```python
from build123d import *

# Parameters (mm, degrees)
F0_R     = 1.5
F1_DEPTH = 20
F2_SIZE  = 0.5
F0_R_2   = 2.75
F3_DEPTH = 2.5
F4_SIZE  = 0.25
F6_DEPTH = 1.3


with BuildPart() as f1:
    # F0 (on Top) → F1 (new body)
    with BuildSketch(Plane.XY):
        Circle(F0_R)
    extrude(amount=-F1_DEPTH)

    # F2
    f2_edges = [f1.edges().sort_by_distance(p)[0] for p in [
        (-1.5, 0, -20),
    ]]
    chamfer(f2_edges, length=F2_SIZE)

    # F0 (on Top) → F3 (join)
    with BuildSketch(Plane.XY):
        Circle(F0_R_2)
        Circle(F0_R, mode=Mode.SUBTRACT)
        Circle(F0_R)
    extrude(amount=F3_DEPTH)

    # F4
    f4_edges = [f1.edges().sort_by_distance(p)[0] for p in [
        (-2.75, 0, 2.5),
        (-2.75, 0, 0),
    ]]
    chamfer(f4_edges, length=F4_SIZE)

    # F5 (on face) → F6 (cut)
    with BuildSketch(Plane.XY.offset(2.5)):
        Polygon((0.75963, -1.281313), (1.489464, 0.017202), (0.729835, 1.298515), (-0.75963, 1.281313), (-1.489464, -0.017202), (-0.729835, -1.298515), align=None)
    extrude(amount=-F6_DEPTH, mode=Mode.SUBTRACT)


solid = f1.part
```
The listing builds one solid part. Answer for the finished solid, in the listing's coordinates (mm). A direction names the side the tool comes from. Give positions to 0.01 mm unless a question says otherwise; leave off trailing zeros. Order: outer loops, then holes, each group sorted by start corner. A loop starts at its lowest first (then second) coordinate and runs counter-clockwise, first axis right, second up. Notation, with made-up numbers: M 14,52 L 20,52 A23 cw 20,68 Z; hole C -11,55 d4. An arc over 180 degrees is marked long. Put each result on its own line as item: value. Start each with the question number.
Item 1: The part is cut by section A-A, the plane z = 1. Determine the outline of the cut face in (x, y), and give its area (3 significant figures).
Item 2: The part is cut by section B-B, the plane x = 0. Determine the outline of the cut face in (y, z).
Item 3: Flat-ended cylindrical pins translate along their axes: P1, Ø1.3, axis at x = 0, y = 0.5, coming from the +Z side; P2, Ø2, axis at x = 0, z = -4.5, coming from the +Y side; P3, Ø1.5, axis at y = 1, z = -8, coming from the -X side. Find the tip coordinate at first contact, or state that the pin passes through.
Item 4: The part is cut by section C-C, the plane z = -16.75. Determine the outline of the cut face in (x, y), and give its area (3 significant figures).
Item 5: Which of the six approach directions +Z, -Z, +X, -X, +Y, -Y give full straight-line access (tool end or side, diameter ignored) to faces 5 (the face through (0, 0, -20)), 6 (the face through (0, -2, 0)), 7 (the face through (-1.115, -0.649, 1.859))?
Item 6: For a pull along X with two mould halves and no side action, classify faces 1 (the face through (1.12, -0.64, 1.86)), 2 (the face through (-1.5, 0.07, -9.61)), 3 (the face through (0, 0, 1.2)), 4 (the face through (1.1, -1.1, 2.5)) as +X half, -X half, draft (parallel to the pull), parting line (faces both ways), or undercut.
Item 7: Find the intervals of material crossed by line 1 along X through (y, z) = (-0.1, -13); line 2 along X through (y, z) = (0.75, -5); line 3 along Z through (x, y) = (1.85, 0), in increasing order.
Answer key:
1. outline: C 0,0 d5.5
1. area: 23.8 mm²
2. outline: M -2.75,0.25 L -2.5,0 L -1.5,0 L -1.5,-19.5 L -1,-20 L 1,-20 L 1.5,-19.5 L 1.5,0 L 2.5,0 L 2.75,0.25 L 2.75,2.25 L 2.5,2.5 L 1.29,2.5 L 1.29,1.2 L -1.29,1.2 L -1.29,2.5 L -2.5,2.5 L -2.75,2.25 Z
3. P1: stops at z = 1.2
3. P2: stops at y = 1.5
3. P3: stops at x = -1.48
4. outline: C 0,0 d3
4. area: 7.07 mm²
5. face 5: -Z, +X, -X, +Y, -Y
5. face 6: -Z
5. face 7: +Z
6. face 1: undercut
6. face 2: parting line
6. face 3: undercut
6. face 4: draft
7. line 1: x = -1.5 to 1.5
7. line 2: x = -1.3 to 1.3
7. line 3: z = 0 to 2.5
